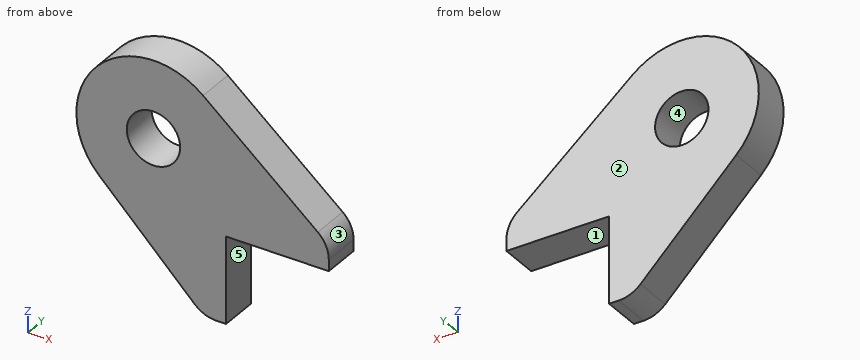
```python
from build123d import *

# Parameters (mm, degrees)
BOSS_EXTRUDE2_DEPTH  = 4.7625
FILLET3_R            = 3.81
M6_CLEARANCE_HOLE3_D = 6.6


with BuildPart() as part:
    # Sketch4 → Boss-Extrude2 (new body)
    with BuildSketch(Plane(origin=(0, 0, 0), x_dir=(1, 0, 0), z_dir=(0, 1, 0))):
        with BuildLine():
            Line((-12.7, -2.013948776), (-12.7, -12.7))
            Line((-12.7, -12.7), (0, -12.7))
            Line((0, -12.7), (0, -15.875))
            Line((0, -15.875), (-15.544691969, -28.965891134))
            ThreePointArc((-15.544691969, -28.965891134), (-28.701038648, -28.117199317), (-28.407157173, -14.936783186))
            Line((-28.407157173, -14.936783186), (-15.452487049, -2.013948776))
            Line((-15.452487049, -2.013948776), (-12.7, -2.013948776))
        make_face()
    extrude(amount=BOSS_EXTRUDE2_DEPTH)

    # Fillet3
    fillet3_edges = [part.edges().sort_by_distance(p)[0] for p in [
        (0, 2.38125, 15.875),
        (-15.452487049, 2.38125, 2.013948776),
    ]]
    fillet(fillet3_edges, radius=FILLET3_R)

    # M6 Clearance Hole3 (through all)
    with Locations(Plane(origin=(0, 4.7625, 0), x_dir=(1, 0, 0), z_dir=(0, 1, 0))):
        with Locations((-21.680256121, -21.680256121)):
            Hole(M6_CLEARANCE_HOLE3_D / 2)


solid = part.part
```
Work out the finished part from the listing and answer in its coordinate system (mm). Face numbers are marked on the shaded views. A direction names the side the tool comes from. Give positions to 0.01 mm unless a question says otherwise; leave off trailing zeros. Order: outer loops, then holes, each group sorted by start corner. A loop starts at its lowest first (then second) coordinate and runs counter-clockwise, first axis right, second up. Notation, with made-up numbers: M -20,11.5 L 37,11.5 A11 cw 37,28.5 Z; hole C 27.5,41.5 d4. An arc over 180 degrees is marked long. Return JSON: item names as keys, results as strings.
1) Straight lines are drawn through the part: line 1 along Z through (x, y) = (-20.5, 0.6); line 2 along X through (y, z) = (0.3, 19.5); line 3 along Z through (x, y) = (-16.5, 0.4). For each, find the intervals that lie inside material, in ascending order. Write a range as [from, to].
Resolved:
{"line 1": "[7.05, 18.6], [24.76, 31.13]", "line 2": "[-30.95, -24.16], [-19.2, -4.3]", "line 3": "[3.06, 29.67]"}
2) A tool of negligible diameter and unlimited length cuts with its end or side. For the marked faces 1 and 2, from which of +Z, -Z, +X, -X, +Y, -Y can it reach the whole face along a straight path? Write none if from no direction.
Resolved:
{"face 1": "-Z, +X, +Y, -Y", "face 2": "+Z, -Z, +X, -X, +Y"}
3) Each of these flat-tipped pins is pushed along its axis until it touches: pin 1 (2 mm diameter, centred on x = -15, y = 4, fed in from +Z); pin 2 (2 mm diameter, centred on x = -19.5, y = 2.5, fed in from -Z). Where does it stop, or does it pass through?
Resolved:
{"pin 1": "z = 29.33", "pin 2": "z = 5.05"}
4) Section D-D, the plane z = 10 is taken. Write down the section's boundary in (x, y).
Resolved:
{"outline": "M -23.46,0 L -12.7,0 L -12.7,4.76 L -23.46,4.76 Z"}
5) For a pull along Z with two mould halves and no side action, classify the marked faces 3, 4 and 5 as +Z half, -Z half, draft (parallel to the pull), parting line (faces both ways), or undercut.
Resolved:
{"face 3": "+Z half", "face 4": "undercut", "face 5": "draft"}
6) Section A-A, the plane z = 23 is taken. Write down the section's boundary in (x, y).
Resolved:
{"outline": "M -31.11,0 L -24.7,0 L -24.7,4.76 L -31.11,4.76 Z; M -18.66,0 L -8.46,0 L -8.46,4.76 L -18.66,4.76 Z"}
7) Section B-B, the plane x = -24.5 is taken. Write down the section's boundary in (y, z).
Resolved:
{"outline": "M 0,11.04 L 4.76,11.04 L 4.76,19.97 L 0,19.97 Z; M 0,23.39 L 4.76,23.39 L 4.76,30.78 L 0,30.78 Z"}
